from build123d import *

# Parameters (mm, degrees)
SKETCH1_R           = 12.5
BOSS_EXTRUDE1_DEPTH = 18
BOSS_EXTRUDE2_START = -4.5
SKETCH2_R           = 25
BOSS_EXTRUDE2_DEPTH = 9
CUT_EXTRUDE1_DEPTH  = 19


with BuildPart() as part:
    # Sketch1 → Boss-Extrude1 (new body)
    with BuildSketch(Plane.XY):
        with Locations((0, -0.049046118)):
            Circle(SKETCH1_R)
    extrude(amount=BOSS_EXTRUDE1_DEPTH)

    # Sketch2 → Boss-Extrude2 (add)
    with BuildSketch(Plane.XY.offset(18).offset(BOSS_EXTRUDE2_START)):
        Circle(SKETCH2_R)
    extrude(amount=-BOSS_EXTRUDE2_DEPTH)

    # Sketch3 → Cut-Extrude1 (cut, through all)
    with BuildSketch(Plane.XY.offset(18)):
        with BuildLine():
            Line((-2, 2.03039405), (2, 2.03039405))
            ThreePointArc((2, 2.03039405), (2.85, 0), (2, -2.03039405))
            Line((2, -2.03039405), (-2, -2.03039405))
            ThreePointArc((-2, -2.03039405), (-2.85, 0), (-2, 2.03039405))
        make_face()
    extrude(amount=-CUT_EXTRUDE1_DEPTH, mode=Mode.SUBTRACT)


solid = part.part
Input: part model. Units: mm. Frame: model coordinates. A direction names the side the tool comes from. Give positions to 0.01 mm unless a question says otherwise; leave off trailing zeros. Write each loop counter-clockwise with the first axis right and the second up, starting at its lowest first coordinate (ties: lowest second). Pieces come first, ordered by that corner, then holes. Notation, with made-up numbers: M 12,16 L 34,16 A17 cw 34,37 Z; hole C 57.5,-26.75 d8. An arc over 180 degrees is marked long. Write item = value, one per line. Start each with the question number.
1) First-contact query: pin 1 Ø3 at (x, z) = (-0.5, 9) entering from -Y; pin 2 Ø6 at (y, z) = (17.5, 10.5) entering from +X; pin 3 Ø4 at (y, z) = (4, 8) entering from -X. Flat tips, straight axial feed; report the tip coordinate or a pass-through.
2) Draft query along Y for faces 1 (the cylindrical face through (-2.71, -12.25, 15.72)), 2 (the cylindrical face through (-2.85, -0.03, 9.13)), 3 (the flat face through (0, -3, 18)). Return one class per face: +Y half, -Y half, draft (parallel to the pull), parting line (faces both ways), or undercut.
3) Cut plane B-B on x = 0. Return the cut outline in (y, z).
4) Cut plane A-A on z = 9.5. Return the cut outline in (x, y), then the cut area to 3 significant figures.
5) Material intervals for line 1 along Z through (x, y) = (-8, -19.5); line 2 along X through (y, z) = (-1.5, 16.5); line 3 along X through (y, z) = (17, 7.5), sorted ascending. Write a range as [from, to].
6) Cut plane C-C on y = 10.5. Return the cut outline in (x, z), then the cut area to 3 significant figures.
7) Cut plane D-D on x = 10. Return the cut outline in (y, z).
8) Reachability of faces 4 (the flat face through (0, -2.03, 9)), 5 (the flat face through (5.2, 11.5, 13.5)), 6 (the flat face through (5.2, 11.5, 4.5)) from +Z, -Z, +X, -X, +Y, -Y: full face, straight path, thin tool, end or side. Return the list, or none.
Solved:
q1.pin_1 = -25
q1.pin_2 = 20.37
q1.pin_3 = -24.92
q2.face_1 = parting line
q2.face_2 = undercut
q2.face_3 = draft
q3.outline = M -25,4.5 L -12.55,4.5 L -12.55,0 L -2.03,0 L -2.03,18 L -12.55,18 L -12.55,13.5 L -25,13.5 Z; M 2.03,0 L 12.45,0 L 12.45,4.5 L 25,4.5 L 25,13.5 L 12.45,13.5 L 12.45,18 L 2.03,18 Z
q4.outline = C 0,0 d50; hole M -2,-2.03 L 2,-2.03 A2.85 ccw 2,2.03 L -2,2.03 A2.85 ccw Z
q4.area = 1,940 mm2
q5.line_1 = [4.5, 13.5]
q5.line_2 = [-12.42, -2.42], [2.42, 12.42]
q5.line_3 = [-18.33, 18.33]
q6.outline = M -22.69,4.5 L -6.71,4.5 L -6.71,0 L 6.71,0 L 6.71,4.5 L 22.69,4.5 L 22.69,13.5 L 6.71,13.5 L 6.71,18 L -6.71,18 L -6.71,13.5 L -22.69,13.5 Z
q6.area = 529 mm2
q7.outline = M -22.91,4.5 L -7.55,4.5 L -7.55,0 L 7.45,0 L 7.45,4.5 L 22.91,4.5 L 22.91,13.5 L 7.45,13.5 L 7.45,18 L -7.55,18 L -7.55,13.5 L -22.91,13.5 Z
q8.face_4 = +Z, -Z
q8.face_5 = +Z
q8.face_6 = -Z
